For this review, take the finished solid that the model builds, in its own axes (mm). A direction names the side the tool comes from. Round coordinates to 2 decimals unless told otherwise and drop trailing zeros. Loops run counter-clockwise (first coordinate to the right, second up) from the corner with the lowest first, then second, coordinate; pieces in that order, holes last. Notation, with made-up numbers: (-27.5, -23) -> (-22.5, -23) arc R23 cw to (-22.5, -10) -> close; hole circle Ø10 at (71.25, -6). An arc over 180 degrees is marked (long way). Use one line per item in the form item = value. Start each with the question number.
from build123d import *

# Parameters (mm, degrees)
F0_W      = 101.6
F0_H      = 101.6
F1_DEPTH  = 2.0066
F3_DEPTH  = 17.018
F4_W      = 95.0976
F4_H      = 95.0976
F5_DEPTH  = 17.018
F6_W      = 93.091
F6_H      = 93.091
F7_DEPTH  = 19.0256
F8_W      = 93.091
F8_H      = 2.0066
F9_DEPTH  = 18.8976
F10_W     = 74.1934
F10_H     = 2.0066
F11_DEPTH = 18.8976


with BuildPart() as f1:
    # F0 (on Top) → F1 (new body)
    with BuildSketch(Plane.XY):
        Rectangle(F0_W, F0_H)
    extrude(amount=-F1_DEPTH)

    # F2 (on face) → F3 (join)
    with BuildSketch(Plane.XY):
        Polygon((-50.8, -50.8), (-48.7934, -50.8), (-48.7934, 48.7934), (50.8, 48.7934), (50.8, 50.8), (-50.8, 50.8), align=None)
    extrude(amount=F3_DEPTH)

    # F4 (on face) → F5 (join, through all)
    with BuildSketch(Plane.XY):
        with Locations((3.2512, -3.2512)):
            Rectangle(F4_W, F4_H)
    extrude(amount=F5_DEPTH)

    # F6 (on face) → F7 (cut, through all)
    with BuildSketch(Plane.XY.offset(17.018)):
        with Locations((4.2545, -4.2545)):
            Rectangle(F6_W, F6_H)
    extrude(amount=-F7_DEPTH, mode=Mode.SUBTRACT)

    # F8 (on face) → F9 (join)
    with BuildSketch(Plane.YZ.offset(-42.291)):
        with Locations((-4.2545, -1.0033)):
            Rectangle(F8_W, F8_H)
    extrude(amount=F9_DEPTH)

    # F10 (on face) → F11 (join)
    with BuildSketch(Plane.XZ.offset(-42.291)):
        with Locations((13.7033, -1.0033)):
            Rectangle(F10_W, F10_H)
    extrude(amount=F11_DEPTH)


solid = f1.part
Item 1: Machinability: for faces 1 (the flat face through (-18, 43, 17.018)), 2 (the flat face through (3, 44.298, 8)), 3 (the flat face through (-50.8, 1, 7)), 4 (the flat face through (-42.291, -5, 9)), 5 (the flat face through (-44.298, -4, 8)), which of the approach directions +Z, -Z, +X, -X, +Y, -Y give a long, thin tool a straight path to every point of the face, cutting with its end or side? Answer none if there is none.
Item 2: For P1, Ø8, axis at x = -28, z = 5.5, coming from the -Y side; P2, Ø6, axis at y = 15.5, z = 7.5, coming from the +X side; P3, Ø1, axis at x = 25.5, z = -1, coming from the -Y side, all flat-tipped, find the tip position at first contact; note any pin that passes through.
Item 3: Take a section at A-A on z = 2.5. Give the boundary of the cut face in (x, y), plus the area to 3 significant figures.
Item 4: Take a section at C-C on y = 16.5. Give the boundary of the cut face in (x, z), plus the area to 3 significant figures.
Item 5: Take a section at B-B on x = -15. Give the boundary of the cut face in (y, z), plus the area to 3 significant figures.
Item 6: Wall thickness on line 1 (Y direction, x = -5, z = 11.75); line 2 (X direction, y = -26, z = 12); line 3 (Z direction, x = -11.5, y = 26.5): over which ranges is each line inside the solid? List them lowest first.
Item 7: Draft analysis for pull direction Y (two halves, no side actions). For faces 6 (the flat face through (1, 50.8, 7)), 7 (the flat face through (-21, 47, 0)), 8 (the flat face through (50.8, 44, 4)), state which applies: +Y half, -Y half, draft (parallel to the pull), parting line (faces both ways), or undercut.
Results:
q1.face_1 = +Z, +X, -X, +Y, -Y
q1.face_2 = +Z, +X
q1.face_3 = +Z, -Z, -X, +Y, -Y
q1.face_4 = +Z, +X, -Y
q1.face_5 = +Z, -Y
q2.P1 = 42.29
q2.P2 = -42.29
q2.P3 = 23.39
q3.outline = (-50.8, -50.8) -> (-48.79, -50.8) -> (-48.79, 48.79) -> (50.8, 48.79) -> (50.8, 50.8) -> (-50.8, 50.8) -> close; (-44.3, -50.8) -> (-42.29, -50.8) -> (-42.29, 42.29) -> (50.8, 42.29) -> (50.8, 44.3) -> (-44.3, 44.3) -> close
q3.area = 781 mm2
q4.outline = (-50.8, -2.01) -> (-23.39, -2.01) -> (-23.39, 0) -> (-42.29, 0) -> (-42.29, 17.02) -> (-44.3, 17.02) -> (-44.3, 0) -> (-48.79, 0) -> (-48.79, 17.02) -> (-50.8, 17.02) -> close
q4.area = 123 mm2
q5.outline = (23.39, -2.01) -> (50.8, -2.01) -> (50.8, 17.02) -> (48.79, 17.02) -> (48.79, 0) -> (44.3, 0) -> (44.3, 17.02) -> (42.29, 17.02) -> (42.29, 0) -> (23.39, 0) -> close
q5.area = 123 mm2
q6.line_1 = 42.29 to 44.3, 48.79 to 50.8
q6.line_2 = -50.8 to -48.79, -44.3 to -42.29
q6.line_3 = -2.01 to 0
q7.face_6 = +Y half
q7.face_7 = undercut
q7.face_8 = draft
